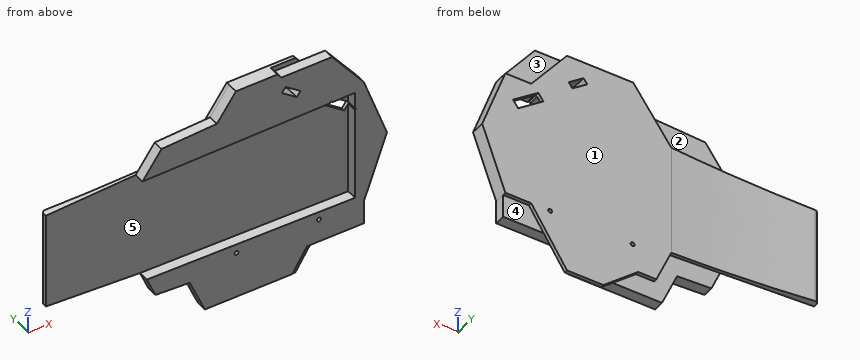
from build123d import *

# Parameters (mm, degrees)
EXTRUDE_1_DEPTH          = 2
EXTRUDE_2_DEPTH          = 2
CUT_EXTRUDE_3_DEPTH      = 202.869395429
CUT_EXTRUDE_3_DEPTH_BACK = 202.869395429
FILLET_1_R               = 2
EXTRUDE_4_DEPTH          = 6
HOLE_WIZARD_4_40_2_D     = 2.2606
CUT_EXTRUDE_7_DEPTH      = 202.98824919


with BuildPart() as part:
    # 草图2 → 凸台-拉伸1 (new body)
    with BuildSketch(Plane(origin=(0, 0, 0), x_dir=(1, 0, 0), z_dir=(0, 1, 0))):
        Polygon((141.821582241, 68.082690978), (121.161879345, 68.082690978), (101.35099463, 51.608897425), (91.039832206, 51.608897425), (82.527346571, 31.825074964), (0, 27.5), (0, -27.5), (82.527346571, -31.825074964), (104.14664553, -61.917309022), (141.821582241, -61.917309022), (162.133732132, -36.18552755), (176.829545061, -36.18552755), (190, 0), (176.829545061, 36.18552755), (162.133732132, 36.18552755), align=None)
    extrude(amount=EXTRUDE_1_DEPTH)

    # 草图6 → 凸台-拉伸2 (add)
    with BuildSketch(Plane(origin=(0, 2, 0), x_dir=(1, 0, 0), z_dir=(0, 1, 0))):
        Polygon((82.527346571, 31.825074964), (82.527346571, -31.825074964), (0, -27.5), (0, 27.5), align=None)
    extrude(amount=EXTRUDE_2_DEPTH)

    # 草图7 → 切除-拉伸3 (cut, two sides: drawn at the far end of the back side and taken through both)
    with BuildSketch(Plane.XY.offset(-CUT_EXTRUDE_3_DEPTH_BACK)):
        with BuildLine():
            Line((82.527346571, 2), (82.527346571, 30.740821148))
            Line((82.527346571, 30.740821148), (0, 4))
            add(Edge.make_bspline(
                [(82.527346571, 2), (41.215261335, 1.001172546), (0, 4)],
                knots=[0, 0, 0, 1, 1, 1], degree=2))
        make_face()
    extrude(amount=CUT_EXTRUDE_3_DEPTH + CUT_EXTRUDE_3_DEPTH_BACK, mode=Mode.SUBTRACT)

    # 圆角1
    fillet_1_edges = [part.edges().sort_by_distance(p)[0] for p in [
        (0, 4, 13.75),
    ]]
    fillet(fillet_1_edges, radius=FILLET_1_R)

    # 草图13 → 凸台-拉伸4 (add)
    with BuildSketch(Plane.XZ):
        Polygon((53.501507434, -30.303895193), (58.412275987, -41.716986195), (77.926898746, -42.739704237), (86.484415452, -62.62818317), (136.164724768, -62.62818317), (144.584081331, -49.40685536), (176.829545061, -49.40685536), (176.829545061, -36.18552755), (190, 0), (176.829545061, 36.18552755), (158.743204348, 59.097615602), (130.016377906, 59.097615602), (127.790568727, 61.917309022), (104.14664553, 61.917309022), (93.336996051, 46.871191993), (61.845926158, 45.220814953), (51.036276678, 30.174697924), (171.852914921, 31.825074964), (171.852914921, -31.825074964), align=None)
    extrude(amount=EXTRUDE_4_DEPTH)

    # #4-40 螺纹孔2 (through all)
    with Locations(Plane(origin=(0, 2, 0), x_dir=(1, 0, 0), z_dir=(0, 1, 0))):
        with Locations((151.351021218, 36.159959894), (104.497931561, 36.159959894)):
            Hole(HOLE_WIZARD_4_40_2_D / 2)

    # 草图18 → 切除-拉伸7 (cut, through all)
    with BuildSketch(Plane(origin=(0, 2, 0), x_dir=(1, 0, 0), z_dir=(0, 1, 0))):
        Polygon((169.563862496, -18.125868021), (155.218286362, -28.471875769), (158.085778721, -32.447885738), (172.431354854, -22.101877989), align=None)
        Polygon((130.302091903, -49.564637909), (132.361562224, -52.420260001), (140.814695434, -46.323873151), (138.755225113, -43.468251059), align=None)
    extrude(amount=-CUT_EXTRUDE_7_DEPTH, mode=Mode.SUBTRACT)


solid = part.part
Work out the finished part from the listing and answer in its coordinate system (mm). Face numbers are marked on the shaded views. A direction names the side the tool comes from. Coordinates: 2 decimals unless noted, no trailing zeros. Write each loop counter-clockwise with the first axis right and the second up, starting at its lowest first coordinate (ties: lowest second). Pieces come first, ordered by that corner, then holes. Notation, with made-up numbers: M -18,17.25 L 16,17.25 A22 ccw 16,34.25 Z; hole C -33.5,45 d11. An arc over 180 degrees is marked long. Answer as CSV lines item,"result". Start each with the question number.
Item 1: Section B-B on x = 97.5 is taken. Write down the section's boundary in (y, z).
Item 2: Section A-A on y = -4.5 is taken. Give the number of separate pieces and of enclosed holes in the cut face, and give its area (3 significant figures).
Item 3: Determine the mould class of the marked faces 4 and 5 for opening direction Z: released by +Z, released by -Z, zero draft, split by the parting line, or undercut.
Item 4: A tool of negligible diameter and unlimited length cuts with its end or side. For the marked faces 1, 2 and 3, from which of +Z, -Z, +X, -X, +Y, -Y can it reach the whole face along a straight path? Write none if from no direction.
Item 5: Section C-C on x = 174.5 is taken. Write down the section's boundary in (y, z), and give its area (3 significant figures).
Item 6: Consider L1, parallel to Y at x = 125, z = -59.5; L2, parallel to Y at x = 157, z = -21.5; L3, parallel to Z at x = 120, y = -0.75. Determine where each line is inside the solid, lowest interval first.
Item 7: Section D-D on x = 148 is taken. Write down the section's boundary in (y, z), and give its area (3 significant figures).
Item 8: Flat-ended cylindrical pins translate along their axes: P1, Ø25, axis at x = 167, z = 50.5, coming from the +Y side; P2, Ø2.5, axis at x = 104.5, z = -36.16, coming from the +Y side; P3, Ø5, axis at y = -2, z = -44.5, coming from the +X side; P4, Ø1.4, axis at x = 151.35, z = -36.16, coming from the -Y side. Find the tip coordinate at first contact, or state that the pin passes through.
Checks:
1,outline,"M -6,-62.63 L 0,-62.63 L 0,-51.61 L 2,-51.61 L 2,52.67 L -6,52.67 L -6,30.81 L 0,30.81 L 0,-30.87 L -6,-30.87 Z"
2,separate pieces,"1"
2,enclosed holes,"3"
2,area,"6,240 mm²"
3,face 4,"zero draft"
3,face 5,"undercut"
4,face 1,"+Z, -Z, +X, +Y"
4,face 2,"+Z, -X, +Y"
4,face 3,"+Z, +X, +Y"
5,outline,"M -6,-49.41 L 0,-49.41 L 0,-36.19 L 2,-36.19 L 2,36.19 L 0,36.19 L 0,39.14 L -6,39.14 Z"
5,area,"676 mm²"
6,L1,"y = -6 to 2"
6,L2,"y = 0 to 2"
6,L3,"z = -62.63 to -31.16, 31.12 to 61.92"
7,outline,"M -6,-49.41 L 0,-49.41 L 0,-58.38 L 2,-58.38 L 2,54.09 L 0,54.09 L 0,59.1 L -6,59.1 L -6,31.5 L 0,31.5 L 0,-31.52 L -6,-31.52 Z"
7,area,"498 mm²"
8,P1,"stops at y = 0"
8,P2,"stops at y = 2"
8,P3,"stops at x = 176.83"
8,P4,"passes through"
